Autodesk Inventor part; units mm, degrees
ref_plane "Work Plane1" through (0, 0, -15) normal (0, 0, 1) x (1, 0, 0)
ref_plane "YZ Plane" through (0, 0, 0) normal (1, 0, 0) x (0, 1, 0)
ref_plane "XZ Plane" through (0, 0, 0) normal (0, 1, 0) x (-1, 0, 0)
sketch "Sketch1" plane through (0, 0, 0) normal (0, 0, 1) x (1, 0, 0)
  line L0 (0, 0) -> (25, 0)
  line L1 (25, 0) -> (25, 40)
  line L2 (25, 40) -> (0, 40)
  line L3 (0, 40) -> (0, 0)
  dimension "d1" = 25
  dimension "d2" = 40
  dimension "d3" = 25
extrude "Extrusion1" add sketch "Sketch1" against normal blind 30
sketch "Sketch2" plane through (25, 0, 0) normal (1, 0, 0) x (0, 0, -1)
  line L0 (0, 0) -> (30, 0)
  circle A0 centre (15, 6.56) radius 2.46
extrude "Extrusion2" cut sketch "Sketch2" against normal blind 30
sketch "Sketch3" plane through (0, 0, 0) normal (-1, 0, 0) x (0, 0, 1)
  line L0 (0, 0) -> (-30, 0)
  line L1 (-25.05, 0) -> (-4.95, 0)
  line L2 (-4.95, 0) -> (-4.95, 33.12)
  line L3 (-4.95, 33.12) -> (-25.05, 33.12)
  line L4 (-25.05, 33.12) -> (-25.05, 0)
  dimension "d11" = 20.1
extrude "Extrusion3" cut sketch "Sketch3" against normal blind 20
sketch "Sketch4" plane through (0, 0, 0) normal (0, -1, 0) x (1, 0, 0)
  line L0 (20, -4.95) -> (20, -25.05)
  line L1 (20, -15) -> (25, -15)
  line L2 (25, 0) -> (25, -30)
  line L3 (20, -8.025) -> (25, -8.025)
  line L4 (25, -8.025) -> (25, -21.975)
  line L5 (25, -21.975) -> (20, -21.975)
  line L6 (20, -21.975) -> (20, -8.025)
  line L7 (20, -8.025) -> (25, -21.975) construction
  line L8 (25, -8.025) -> (20, -21.975) construction
  line L9 (25, -12.54) -> (25, -17.46)
  point P0 (0, 0)
  point P1 (22.5, -15)
  dimension "d14" = 13.95
extrude "Extrusion4" add sketch "Sketch4" along normal blind 15
sketch "Sketch5" plane through (20, 0, 0) normal (-1, 0, 0) x (0, 0, 1)
  circle A0 centre (-15, 6.56) radius 2.46
  circle A1 centre (-15, 6.56) radius 4.7025
  circle A2 centre (-15, 6.56) radius 2.46
  circle A3 centre (-15, 6.56) radius 2.46
  point P0 (0, 0)
  dimension "d17" = 9.405
extrude "Extrusion5" cut sketch "Sketch5" against normal blind 2.1
sketch "Sketch6" plane through (25, 0, 0) normal (1, 0, 0) x (0, 0, -1)
  circle A0 centre (15, 6.56) radius 4.7025
  line L0 (15, 6.56) -> (15, 23.56)
  circle A1 centre (15, 23.56) radius 2.46
  point P0 (0, 0)
  dimension "d20" = 17
  dimension "d21" = 4.92
extrude "Extrusion6" cut sketch "Sketch6" against normal blind 10 contours A1
sketch "Sketch7" plane through (20, 0, 0) normal (-1, 0, 0) x (0, 0, 1)
  circle A0 centre (-15, 23.56) radius 2.46
  circle A1 centre (-15, 23.56) radius 4.7025
  point P0 (0, 0)
  dimension "d24" = 9.405
extrude "Extrusion7" cut sketch "Sketch7" against normal blind 2.1
sketch "Sketch9" plane through (25, 0, 0) normal (1, 0, 0) x (0, 0, -1)
  circle A0 centre (15, 6.56) radius 2.46
  circle A1 centre (15, 6.56) radius 2.46
  circle A2 centre (15, 23.56) radius 2.46
  circle A3 centre (15, 23.56) radius 2.46
  line L0 (30, 40) -> (30, 0)
  line L1 (30, 0) -> (30, 40)
  line L2 (30, 40) -> (0, 40)
  line L3 (0, 40) -> (0, 0)
  line L4 (0, 0) -> (8.025, 0)
  line L5 (21.975, 0) -> (21.975, -15)
  line L6 (21.975, -15) -> (8.025, -15)
  line L7 (8.025, -15) -> (8.025, 0)
  line L8 (0, 0) -> (8.025, 0)
  line L9 (21.975, 0) -> (30, 0)
extrude "Extrusion8" add sketch "Sketch9" along normal blind 5
sketch "Sketch10" plane through (0, 40, 0) normal (0, 1, 0) x (1, 0, 0)
  line L0 (0, 30) -> (30, 30)
  line L1 (30, 0) -> (0, 0)
  line L2 (0, 30) -> (30, 30)
  line L3 (30, 30) -> (30, 0)
  line L4 (30, 0) -> (0, 0)
  line L5 (0, 0) -> (0, 30)
extrude "Extrusion9" add sketch "Sketch10" along normal blind 30
sketch "Sketch12" plane through (30, 0, 0) normal (1, 0, 0) x (0, 0, -1)
  circle A0 centre (15, 6.56) radius 2.46
  line L0 (15, 6.56) -> (15, 15.06)
  circle A1 centre (15, 15.06) radius 2.525
  point P0 (0, 0)
  dimension "d31" = 8.5
  dimension "d33" = 5.05
extrude "Extrusion10" cut sketch "Sketch12" against normal blind 30 contours A1
sketch "Sketch14" plane through (0, 0, 0) normal (0, 0, 1) x (1, 0, 0)
  line L0 (30, 70) -> (0, 70)
  line L1 (0, 70) -> (0, 85)
  line L2 (-15, 100) -> (-23, 100)
  line L3 (30, 0) -> (30, 70)
  line L4 (30, 118) -> (30, 70)
  arc A0 (0, 85) -> (-15, 100) centre (-15, 85) ccw
  line L5 (30, 105) -> (30, 100)
  line L6 (-23, 133) -> (15, 133)
  line L7 (-18, 130.5) -> (-23, 133)
  line L8 (-18, 130.5) -> (-13, 116.5)
  line L9 (-18, 102.5) -> (-23, 100)
  line L10 (-18, 102.5) -> (-13, 116.5)
  line L11 (30, 118) -> (15, 133)
  point P0 (0, 0)
  point P1 (0, 100)
  dimension "d47" = 30
  dimension "d54" = 15
extrude "Extrusion12" add sketch "Sketch14" against normal blind 30
sketch "Sketch15" plane through (0, 0, -25.05) normal (-1, 0, 0) x (0, 0, 1)
  line L0 (0, 33.12) -> (20.1, 33.12)
  line L1 (20.1, 33.12) -> (20.1, 0)
  line L2 (0, 33.12) -> (20.1, 33.12)
  line L3 (20.1, 33.12) -> (20.1, 31.1)
  line L4 (20.1, 31.1) -> (0, 31.1)
  line L5 (0, 31.1) -> (0, 33.12)
  point P0 (25.05, 0)
  dimension "d57" = 2.02
extrude "Extrusion13" add sketch "Sketch15" against normal blind 20
sketch "Sketch21" plane through (0, 0, 0) normal (0, 0, 1) x (1, 0, 0)
  arc A0 (0, 85) -> (-15, 100) centre (-15, 85) ccw
  arc A1 (0, 85) -> (-15, 100) centre (-15, 85) ccw
  line L0 (-15, 100) -> (-23, 100)
  line L1 (-15, 100) -> (-23, 100)
  line L2 (-23, 100) -> (-18, 102.5)
  line L3 (-23, 100) -> (-18, 102.5)
  line L4 (-18, 102.5) -> (-13, 116.5)
  line L5 (-18, 102.5) -> (-13, 116.5)
  line L6 (-13, 116.5) -> (-18, 130.5)
  line L7 (-13, 116.5) -> (-18, 130.5)
  line L8 (-18, 130.5) -> (-23, 133)
  line L9 (-18, 130.5) -> (-23, 133)
  line L10 (-23, 133) -> (15, 133)
  line L11 (-23, 133) -> (15, 133)
  line L12 (15, 133) -> (30, 118)
  line L13 (15, 133) -> (30, 118)
  line L14 (0, 85) -> (30, 85)
  line L15 (30, 85) -> (30, 118)
  point P0 (0, 0)
extrude "Extrusion14" add sketch "Sketch21" along normal blind 30
ref_plane "Work Plane1" through (0, 0, -15) normal (0, 0, 1) x (1, 0, 0)
mirror "Mirror1" about plane through (0, 0, -15) normal (0, 0, 1) of "Extrusion14"
properties part number "28mm_x_90mm"
Geometry check sheet. Reference: the model listing, model coordinates, mm. A direction names the side the tool comes from. Give positions to 0.01 mm unless a question says otherwise; leave off trailing zeros. Loops run counter-clockwise (first coordinate to the right, second up) from the corner with the lowest first, then second, coordinate; pieces in that order, holes last. Notation, with made-up numbers: (59.5, 28.5) -> (105.5, 28.5) arc R6 cw to (105.5, 39.5) -> close; hole circle Ø10 at (65, 20). An arc over 180 degrees is marked (long way). Answer in a Markdown table with one row per item. Add a question column.
1) Material ranges on probe 1 along X at (y, z) = (40.5, -10.5); probe 2 along Y at (x, z) = (21.1, -15) (1 decimal); probe 3 along Z at (x, y) = (1.5, 70), recorded low to high. Write a range as from..to.
2) Cross-section at B-B on x = -20. Record the boundary of the cut face in (y, z), and give its area (3 significant figures).
3) Draft check along Y on faces 1 (the face through (10, 109, -60)), 2 (the face through (15, 85, 15)), 3 (the face through (21.035, 7.973, -10.515)). Enter one of: pulls with the +Y half, pulls with the -Y half, needs draft (parallel to the pull), parting line crosses it, or undercut.
4) Cross-section at D-D on x = 18. Record the boundary of the cut face in (y, z), and give its area (3 significant figures).
5) Gauge pin test, flat ends, axial feed: P1, Ø4, axis at y = 23.56, z = -15, coming from the -X side (3 decimals); P2, Ø24, axis at y = 59, z = -15, coming from the -X side; P3, Ø6, axis at x = 14.5, y = 12.5, coming from the -Z side; P4, Ø3, axis at y = 22, z = -13.5, coming from the -X side. Record the tip position at first contact, or that the pin passes through.
6) Cross-section at C-C on y = 23.56. Record the boundary of the cut face in (x, z), and give its area (3 significant figures).
7) Set-up check for faces 4 (the face through (22.1, 21.5, -13)), 5 (the face through (10, 16, -25.05)), 6 (the face through (15, 43, 0)), 7 (the face through (-19, 100, -14)), 8 (the face through (-21, 132, -14)): record each of +Z, -Z, +X, -X, +Y, -Y from which the full face is reachable in a straight line by a thin tool's end or side.
8) Cross-section at A-A on z = -15. State how many separate pieces and enclosed holes the cut face has, and give its area (3 significant figures).
Outcome:
| question | item | result |
|---|---|---|
| 1 | probe 1 | x = 0..30 |
| 1 | probe 2 | y = -15..1.9, 11.3..12.5, 17.6..18.9, 28.3..126.9 |
| 1 | probe 3 | z = -30..0 |
| 2 | outline | (100, -60) -> (101.5, -60) -> (101.5, 30) -> (100, 30) -> close; (131.5, -60) -> (133, -60) -> (133, 30) -> (131.5, 30) -> close |
| 2 | area | 270 mm^2 |
| 3 | face 1 | needs draft |
| 3 | face 2 | pulls with the -Y half |
| 3 | face 3 | undercut |
| 4 | outline | (0, -30) -> (85, -30) -> (85, -60) -> (130, -60) -> (130, 30) -> (85, 30) -> (85, 0) -> (0, 0) -> (0, -4.95) -> (31.1, -4.95) -> (31.1, -25.05) -> (0, -25.05) -> close |
| 4 | area | 5,970 mm^2 |
| 5 | P1 | passes through |
| 5 | P2 | stops at x = 0 |
| 5 | P3 | stops at z = -30 |
| 5 | P4 | stops at x = 22.1 |
| 6 | outline | (0, -30) -> (30, -30) -> (30, -17.46) -> (22.1, -17.46) -> (22.1, -19.7) -> (20, -19.7) -> (20, -25.05) -> (0, -25.05) -> close; (0, -4.95) -> (20, -4.95) -> (20, -10.3) -> (22.1, -10.3) -> (22.1, -12.54) -> (30, -12.54) -> (30, 0) -> (0, 0) -> close |
| 6 | area | 439 mm^2 |
| 7 | face 4 | -X |
| 7 | face 5 | -X, -Y |
| 7 | face 6 | +Z, +X, -X, -Y |
| 7 | face 7 | +Z, -Z, -X, -Y |
| 7 | face 8 | +Z, -Z, -X |
| 8 | separate pieces | 4 |
| 8 | enclosed holes | 0 |
| 8 | area | 3,820 mm^2 |
